Source: CAD feature listing. Evaluate the final solid. Frame: model axes, mm. A direction names the side the tool comes from. Coordinates: 2 decimals unless noted, no trailing zeros. Order: outer loops, then holes, each group sorted by start corner. A loop starts at its lowest first (then second) coordinate and runs counter-clockwise, first axis right, second up.
```python
from build123d import *

# Parameters (mm, degrees)
F1_DEPTH = 25.4
F3_D     = 6.5278
F7_DEPTH = 12.7
F8_R     = 12.7
F9_D     = 25.4


with BuildPart() as f1:
    # F0 (on Top) → F1 (new body, symmetric)
    with BuildSketch(Plane.XY):
        with BuildLine():
            Line((0, 50.8), (-28.3980633142, 50.8))
            ThreePointArc((-28.3980633142, 50.8), (-38.1, 25.4), (-28.3980633142, 0))
            Line((-28.3980633142, 0), (0, 0))
            Line((0, 0), (0, 12.7))
            ThreePointArc((0, 12.7), (-12.7, 25.4), (0, 38.1))
            Line((0, 38.1), (0, 50.8))
        make_face()
    extrude(amount=F1_DEPTH, both=True)

    # F3 (through all)
    with Locations(Plane.YZ):
        with Locations((6.35, 12.7), (44.45, 12.7), (44.45, -12.7), (6.35, -12.7)):
            Hole(F3_D / 2)

    # F6 (on plane+point) → F7 (cut)
    with BuildSketch(Plane.YZ.offset(-38.1)):
        Polygon((0.850738686, 15.875), (0.850738686, 9.525), (6.35, 6.35), (11.849261314, 9.525), (11.849261314, 15.875), (6.35, 19.05), align=None)
        Polygon((38.950738686, 15.875), (38.950738686, 9.525), (44.45, 6.35), (49.949261314, 9.525), (49.949261314, 15.875), (44.45, 19.05), align=None)
        Polygon((44.45, -6.35), (38.950738686, -9.525), (38.950738686, -15.875), (44.45, -19.05), (49.949261314, -15.875), (49.949261314, -9.525), align=None)
        Polygon((6.35, -6.35), (0.850738686, -9.525), (0.850738686, -15.875), (6.35, -19.05), (11.849261314, -15.875), (11.849261314, -9.525), align=None)
    extrude(amount=F7_DEPTH, mode=Mode.SUBTRACT)

    # F8
    f8_edges = [f1.edges().sort_by_distance(p)[0] for p in [
        (-14.199032, 0, 25.4),
        (-14.199032, 50.8, 25.4),
        (-14.199032, 0, -25.4),
        (-14.199032, 50.8, -25.4),
    ]]
    fillet(f8_edges, radius=F8_R)

    # F9 (through all)
    with Locations(Plane.YZ):
        with Locations((25.4, 0)):
            Hole(F9_D / 2)


solid = f1.part
```
1. Ray query, line 1 (Y direction, x = -28, z = 0); line 2 (Z direction, x = -7, y = 44.45); line 3 (Z direction, x = -32.5, y = 39.5). Return the intervals inside material, ascending.
Findings:
line 1: y = 0 to 12.7, 38.1 to 50.8
line 2: z = -23.7 to -15.96, -9.44 to 9.44, 15.96 to 23.7
line 3: z = -25.32 to -16.19, -9.21 to 9.21, 16.19 to 25.32
2. Access query for faces 1 (the face through (-31, 11.849, 13)), 2 (the face through (-14.22, 47.18, -21.58)). Directions: +Z, -Z, +X, -X, +Y, -Y. A direction counts if a zero-diameter tool reaches every point of the face in a straight line with its end or side. Return the directions, or none.
Findings:
face 1: -X
face 2: -Z, +X, -X, +Y
3. Section query A-A on x = -11. Return loops of the section in (y, z).
Findings:
outline: (0, -12.7) arc R12.7 ccw to (12.7, -25.4) - (19.05, -25.4) - (19.05, -11) arc R12.7 cw to (19.05, 11) - (19.05, 25.4) - (12.7, 25.4) arc R12.7 ccw to (0, 12.7) - close; (31.75, -25.4) - (38.1, -25.4) arc R12.7 ccw to (50.8, -12.7) - (50.8, 12.7) arc R12.7 ccw to (38.1, 25.4) - (31.75, 25.4) - (31.75, 11) arc R12.7 cw to (31.75, -11) - close; hole circle Ø6.53 at (6.35, -12.7); hole circle Ø6.53 at (6.35, 12.7); hole circle Ø6.53 at (44.45, -12.7); hole circle Ø6.53 at (44.45, 12.7)
4. Pin query (flat end, axial travel): P1, Ø8.5, axis at y = 6.35, z = 12.7, coming from the -X side; P2, Ø1.1, axis at x = -27.5, z = -14, coming from the -Y side; P3, Ø8, axis at x = -24.5, y = 7, coming from the -Z side; P4, Ø6, axis at y = 44.45, z = -12.7, coming from the +X side. Return the tip coordinate at first contact, or that it passes through.
Findings:
P1: stops at x = -25.4
P2: stops at y = 0.02
P3: stops at z = -25.29
P4: passes through
5. Draft query along Y for faces 3 (the face through (-13.72, 3.82, 21.78)), 4 (the face through (-14, 50.8, 0)), 5 (the face through (-12.697, 25.121, -15.344)). Return one class per face: released by +Y, released by -Y, zero draft, split by the parting line, or undercut.
Findings:
face 3: released by -Y
face 4: released by +Y
face 5: undercut
6. Section query D-D on z = 11. Return loops of the section in (x, y), plus the area to 3 significant figures.
Findings:
outline: (-37.57, 19.05) arc R38.1 ccw to (-35.61, 11.85) - (-25.4, 11.85) - (-25.4, 9.14) - (0, 9.14) - (0, 12.7) arc R12.7 cw to (-11, 19.05) - close; (-37.57, 31.75) - (-11, 31.75) arc R12.7 cw to (0, 38.1) - (0, 41.66) - (-25.4, 41.66) - (-25.4, 38.95) - (-35.61, 38.95) arc R38.1 ccw to start; (-29.14, 0.85) arc R38.1 ccw to (-28.4, 0) - (0, 0) - (0, 3.56) - (-25.4, 3.56) - (-25.4, 0.85) - close; (-29.14, 49.95) - (-25.4, 49.95) - (-25.4, 47.24) - (0, 47.24) - (0, 50.8) - (-28.4, 50.8) arc R38.1 ccw to start
area: 754 mm2
7. Section query B-B on x = -23. Return loops of the section in (y, z).
Findings:
outline: (0, -12.7) arc R12.7 ccw to (12.7, -25.4) - (38.1, -25.4) arc R12.7 ccw to (50.8, -12.7) - (50.8, 12.7) arc R12.7 ccw to (38.1, 25.4) - (12.7, 25.4) arc R12.7 ccw to (0, 12.7) - close; hole circle Ø6.53 at (6.35, -12.7); hole circle Ø6.53 at (6.35, 12.7); hole circle Ø25.4 at (25.4, 0); hole circle Ø6.53 at (44.45, -12.7); hole circle Ø6.53 at (44.45, 12.7)
8. Section query C-C on z = -3. Return loops of the section in (x, y).
Findings:
outline: (-36.05, 13.06) arc R38.1 ccw to (-28.4, 0) - (0, 0) - (0, 12.7) arc R12.7 cw to (-3, 13.06) - close; (-36.05, 37.74) - (-3, 37.74) arc R12.7 cw to (0, 38.1) - (0, 50.8) - (-28.4, 50.8) arc R38.1 ccw to start
